Model file for the job. Use its own axes, mm. A direction names the side the tool comes from. Coordinates: 2 decimals unless noted, no trailing zeros. Order: outer loops, then holes, each group sorted by start corner. A loop starts at its lowest first (then second) coordinate and runs counter-clockwise, first axis right, second up. Notation, with made-up numbers: (15, 73) -> (55, 73) arc R34 cw to (55, 103) -> close; hole circle Ø4 at (-24, 83.5). An arc over 180 degrees is marked (long way). Write item = value, one per line. Start each with the question number.
Q1. Cut at B-B, the plane x = 40. List the corners of the cut face in (y, z) (1 decimal), plus the area to 3 significant figures.
Q2. Cut at A-A, the plane y = -10.5. List the corners of the cut face in (x, z) (1 decimal), plus the area to 3 significant figures.
Q3. Wall check: line 1 (X direction, y = 7.5, z = 11) (3 decimals); line 2 (Y direction, x = 11.5, z = 15.25); line 3 (Y direction, x = 25, z = 18.5). Give the ranges that are in metal, low to high. Write a range as from..to.
Q4. Flat gauge pins, fed straight in: pin 1 (1.5 mm diameter, centred on x = -6.5, z = 3, fed in from -Y); pin 2 (12 mm diameter, centred on x = 40.5, z = 10.5, fed in from +Y) (3 decimals); pin 3 (3 mm diameter, centred on y = -13, z = 10.5, fed in from -X); pin 4 (6 mm diameter, centred on y = -0.5, z = 5.5, fed in from -X) (3 decimals). Where does each tip first touch, or does it go through?
Q5. Mould opens along X. For faces 1 (the face through (22.225, 9, 11)), 2 (the face through (24, 10.287, 11)), 3 (the face through (45.847, -2, 11)) say: +X half, -X half, draft (parallel to the pull), parting line (faces both ways), or undercut.
Q6. 3-axis set-ups, long thin cutter, end or side, ignore diameter. For faces 4 (the face through (-9.068, 13, 11)), 5 (the face through (-5.41, -14, 11)), 6 (the face through (37, -8.509, 11)), 7 (the face through (36.413, -0.884, 21.716)): which of +Z, -Z, +X, -X, +Y, -Y reach the whole face in a straight line?
Q7. Cut at D-D, the plane y = 5. Give the number of separate pieces and of enclosed holes in the cut face, plus the area to 3 significant figures.
Q8. Cut at C-C, the plane y = 11.5. List the corners of the cut face in (x, z).
from build123d import *

# Parameters (mm, degrees)
F0_W      = 36.83
F0_H      = 17.018
F1_DEPTH  = 22.479
F2_R      = 7.112
F1_FACE_W = 17.018
F1_FACE_H = 8.255
F4_DEPTH  = 27.432
F6_DEPTH  = 16.002
F7_R      = 12.816169
F7_R_2    = 4.7625
F8_DEPTH  = 1.524
F9_R      = 1.524
F10_R     = 1.016
F11_DEPTH = 2.032
F12_W     = 2.54
F12_H     = 5.08
F13_DEPTH = 2.54
F15_DEPTH = 1.143
F16_W     = 2.54
F16_H     = 5.08
F17_DEPTH = 2.54
F19_DEPTH = 8.89
F21_DEPTH = 8.89
F22_R     = 1.324614
F23_DEPTH = 1.9558
F24_R     = 1.419753
F25_DEPTH = 25.4


with BuildPart() as f1:
    # F0 (on Top) → F1 (new body)
    with BuildSketch(Plane.XY):
        with Locations((0, -0.762)):
            Rectangle(F0_W, F0_H)
    extrude(amount=F1_DEPTH)

    # F2
    f2_edges = [f1.edges().sort_by_distance(p)[0] for p in [
        (-18.415, -0.762, 22.479),
        (-18.415, -0.762, 0),
    ]]
    fillet(f2_edges, radius=F2_R)

    # F3 (on face) + F1_face (on face) → F4 (join)
    with BuildSketch(Plane.YZ.offset(18.415)):
        with BuildLine():
            Line((-9.271, 18.582747), (-9.271, 3.896253))
            ThreePointArc((-9.271, 3.896253), (-5.441313, 1.020381), (-0.762, 0))
            ThreePointArc((-0.762, 0), (3.917313, 1.020381), (7.747, 3.896253))
            Line((7.747, 3.896253), (7.747, 18.582747))
            ThreePointArc((7.747, 18.582747), (3.917313, 21.458619), (-0.762, 22.479))
            ThreePointArc((-0.762, 22.479), (-5.441313, 21.458619), (-9.271, 18.582747))
        make_face()
    with BuildSketch(Plane(origin=(18.415, -0.762, 11.2395), x_dir=(0, 1, 0), z_dir=(1, 0, 0))):
        Rectangle(F1_FACE_W, F1_FACE_H)
    extrude(amount=F4_DEPTH)

    # F5 (on face) → F6 (cut)
    with BuildSketch(Plane.YZ.offset(45.847)):
        with BuildLine():
            ThreePointArc((13.335, 20.428588), (-0.762, 28.067), (-14.859, 20.428588))
            Line((-14.859, 20.428588), (-14.859, 2.050412))
            ThreePointArc((-14.859, 2.050412), (-0.762, -5.588), (13.335, 2.050412))
            Line((13.335, 2.050412), (13.335, 20.428588))
        make_face()
        with BuildLine():
            ThreePointArc((-9.271, 18.582747), (-0.762, 22.479), (7.747, 18.582747))
            Line((7.747, 18.582747), (7.747, 3.896253))
            ThreePointArc((7.747, 3.896253), (-0.762, 0), (-9.271, 3.896253))
            Line((-9.271, 3.896253), (-9.271, 18.582747))
        make_face(mode=Mode.SUBTRACT)
        with BuildLine():
            Line((7.747, 3.896253), (7.747, 18.582747))
            ThreePointArc((7.747, 18.582747), (-0.762, 22.479), (-9.271, 18.582747))
            Line((-9.271, 18.582747), (-9.271, 3.896253))
            ThreePointArc((-9.271, 3.896253), (-0.762, 0), (7.747, 3.896253))
        make_face()
        with BuildLine():
            Line((-8.509, 4.185282), (-8.509, 18.293718))
            ThreePointArc((-8.509, 18.293718), (-0.762, 21.717), (6.985, 18.293718))
            Line((6.985, 18.293718), (6.985, 4.185282))
            ThreePointArc((6.985, 4.185282), (-0.762, 0.762), (-8.509, 4.185282))
        make_face(mode=Mode.SUBTRACT)
    extrude(amount=-F6_DEPTH, mode=Mode.SUBTRACT)

    # F7 (on face) → F8 (cut)
    with BuildSketch(Plane.YZ.offset(45.847)):
        with Locations((-0.762, 11.2395)):
            Circle(F7_R)
        with BuildLine():
            ThreePointArc((6.985, 4.185282), (-0.762, 0.762), (-8.509, 4.185282))
            Line((-8.509, 4.185282), (-8.509, 18.293718))
            ThreePointArc((-8.509, 18.293718), (-0.762, 21.717), (6.985, 18.293718))
            Line((6.985, 18.293718), (6.985, 4.185282))
        make_face(mode=Mode.SUBTRACT)
        with BuildLine():
            Line((-8.509, 18.293718), (-8.509, 4.185282))
            ThreePointArc((-8.509, 4.185282), (-0.762, 0.762), (6.985, 4.185282))
            Line((6.985, 4.185282), (6.985, 18.293718))
            ThreePointArc((6.985, 18.293718), (-0.762, 21.717), (-8.509, 18.293718))
        make_face()
        with Locations((-0.762, 11.2395)):
            Circle(F7_R_2, mode=Mode.SUBTRACT)
    extrude(amount=-F8_DEPTH, mode=Mode.SUBTRACT)

    # F9
    f9_edges = [f1.edges().sort_by_distance(p)[0] for p in [
        (44.323, -0.762, 0.762),
        (44.323, -0.762, 21.717),
    ]]
    fillet(f9_edges, radius=F9_R)

    # F10 (on face) → F11 (join)
    with BuildSketch(Plane.YZ.offset(45.847)):
        with Locations((-0.762, 11.2395)):
            Circle(F10_R)
    extrude(amount=F11_DEPTH)

    # F12 (on face) → F13 (join)
    with BuildSketch(Plane.XZ.offset(9.271)):
        with Locations((23.495, 11.2395)):
            Rectangle(F12_W, F12_H)
    extrude(amount=F13_DEPTH)

    # F14 (on face) → F15 (join)
    with BuildSketch(Plane(origin=(0, 7.747, 0), x_dir=(-1, 0, 0), z_dir=(0, 1, 0))):
        with BuildLine():
            Line((-18.415, 0), (11.303, 0))
            ThreePointArc((11.303, 0), (16.331943, 2.083057), (18.415, 7.112))
            Line((18.415, 7.112), (18.415, 15.367))
            ThreePointArc((18.415, 15.367), (16.331943, 20.395943), (11.303, 22.479))
            Line((11.303, 22.479), (-18.415, 22.479))
            Line((-18.415, 22.479), (-18.415, 18.582747))
            Line((-18.415, 18.582747), (-18.415, 3.896253))
            Line((-18.415, 3.896253), (-18.415, 0))
        make_face()
    extrude(amount=F15_DEPTH)

    # F16 (on face) → F17 (join)
    with BuildSketch(Plane(origin=(0, 7.747, 0), x_dir=(-1, 0, 0), z_dir=(0, 1, 0))):
        with Locations((-23.495, 11.2395)):
            Rectangle(F16_W, F16_H)
    extrude(amount=F17_DEPTH)

    # F18 (on face) → F19 (join)
    with BuildSketch(Plane.XZ.offset(9.271)):
        with BuildLine():
            Line((-5.4102, 9.280857), (-5.4102, 13.198143))
            ThreePointArc((-5.4102, 13.198143), (-7.239, 13.9192), (-9.0678, 13.198143))
            Line((-9.0678, 13.198143), (-9.0678, 9.280857))
            ThreePointArc((-9.0678, 9.280857), (-7.239, 8.5598), (-5.4102, 9.280857))
        make_face()
    extrude(amount=F19_DEPTH)

    # F20 (on face) → F21 (join)
    with BuildSketch(Plane(origin=(0, 8.89, 0), x_dir=(-1, 0, 0), z_dir=(0, 1, 0))):
        with BuildLine():
            Line((5.4102, 13.198143), (5.4102, 9.280857))
            ThreePointArc((5.4102, 9.280857), (7.239, 8.5598), (9.0678, 9.280857))
            Line((9.0678, 9.280857), (9.0678, 13.198143))
            ThreePointArc((9.0678, 13.198143), (7.239, 13.9192), (5.4102, 13.198143))
        make_face()
    extrude(amount=F21_DEPTH)

    # F22 (on face) → F23 (join)
    with BuildSketch(Plane(origin=(0, 8.89, 0), x_dir=(-1, 0, 0), z_dir=(0, 1, 0))):
        with Locations((-4.0386, 11.2395)):
            Circle(F22_R)
    extrude(amount=F23_DEPTH)

    # F24 (on face) → F25 (cut)
    with BuildSketch(Plane.XZ.offset(9.271)):
        with Locations((13.843, 20.0025)):
            Circle(F24_R)
        with Locations((13.843, 2.4765)):
            Circle(F24_R)
    extrude(amount=-F25_DEPTH, mode=Mode.SUBTRACT)


solid = f1.part
Here are the results:
q1.outline = (-8.5, 4.2) arc R10.5 ccw to (7, 4.2) -> (7, 18.3) arc R10.5 ccw to (-8.5, 18.3) -> close
q1.area = 292 mm²
q2.outline = (-9.1, 9.3) arc R2.7 ccw to (-5.4, 9.3) -> (-5.4, 13.2) arc R2.7 ccw to (-9.1, 13.2) -> close; (22.2, 8.7) -> (24.8, 8.7) -> (24.8, 13.8) -> (22.2, 13.8) -> close
q2.area = 30.9 mm²
q3.line_1 = -18.415..29.845
q3.line_2 = -9.27..8.89
q3.line_3 = -9.27..7.75
q4.pin_1 = -9.27
q4.pin_2 = 6.985
q4.pin_3 = -9.07
q4.pin_4 = -18.415
q5.face_1 = undercut
q5.face_2 = draft
q5.face_3 = +X half
q6.face_4 = +Z, -Z, -X, +Y
q6.face_5 = +Z, -Z, -Y
q6.face_6 = +Z, -Z, +X, -Y
q6.face_7 = +Z, +X
q7.separate_pieces = 1
q7.enclosed_holes = 2
q7.area = 1,270 mm²
q8.outline = (-9.07, 9.28) arc R2.68 ccw to (-5.41, 9.28) -> (-5.41, 13.2) arc R2.68 ccw to (-9.07, 13.2) -> close
